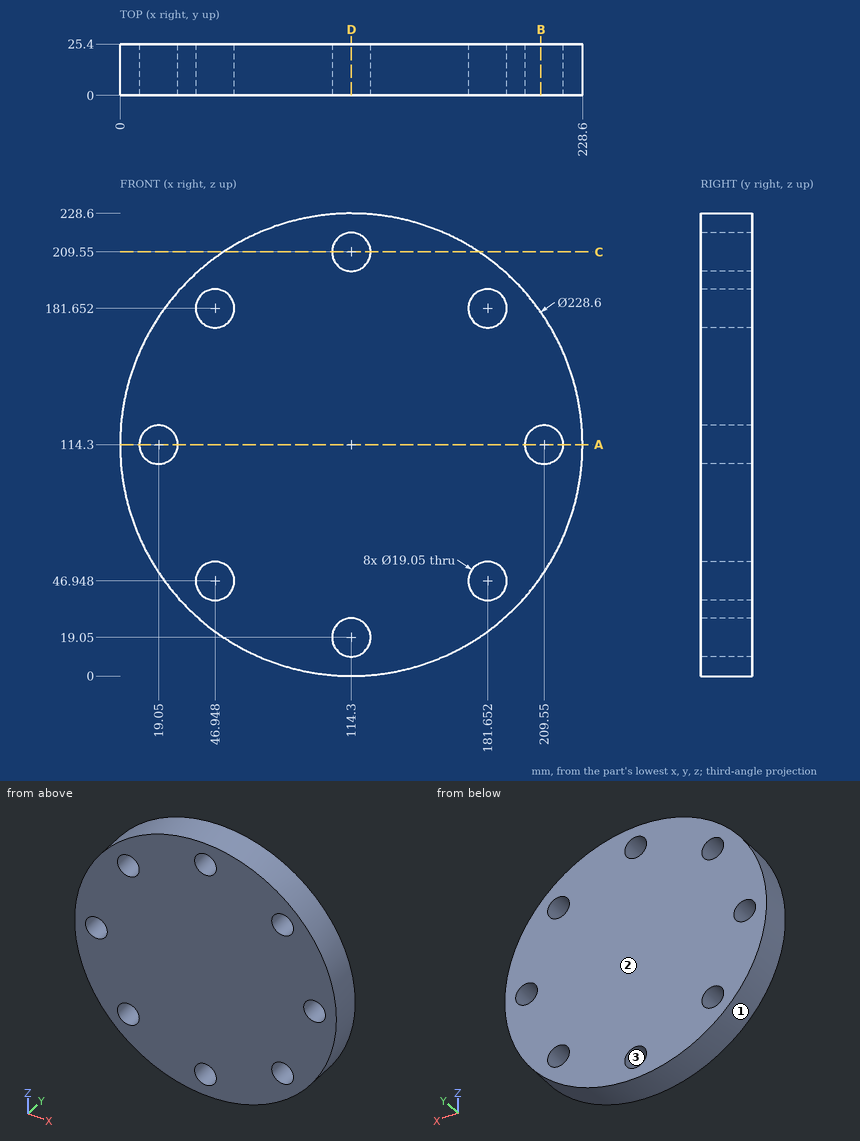
Study the drawing (mm; zero at the part's minimum x, y, z) and answer. Round coordinates to 2 decimals unless told otherwise and drop trailing zeros. Order: outer loops, then holes, each group sorted by start corner. A loop starts at its lowest first (then second) coordinate and runs counter-clockwise, first axis right, second up. Notation, with made-up numbers: M 67,60.25 L 83,60.25 A14 cw 83,82.25 Z; hole C 73,81 d1. An arc over 180 degrees is marked long. One line per item, written item: value.
Q1. Flat-ended cylindrical pins translate along their axes: pin 1 (4 mm diameter, centred on x = 174.5, z = 55.5, fed in from -Y); pin 2 (2 mm diameter, centred on x = 90.5, y = 17.5, fed in from +Z); pin 3 (4 mm diameter, centred on y = 8, z = 152, fed in from +X); pin 4 (10 mm diameter, centred on y = 10, z = 128.5, fed in from -X). Find the tip coordinate at first contact, or state that the pin passes through.
Derived:
pin 1: y = 0
pin 2: z = 226.3
pin 3: x = 222.88
pin 4: x = 0.37
Q2. Straight lines are drawn through the part: line 1 (Z direction, x = 114.3, y = 5.75) (3 decimals); line 2 (Z direction, x = 176, y = 14) (1 decimal); line 3 (X direction, y = 14, z = 212) (1 decimal). For each, find the intervals that lie inside material, in ascending order.
Derived:
line 1: 0 to 9.525, 28.575 to 200.025, 219.075 to 228.6
line 2: 18.1 to 39.3, 54.6 to 174, 189.3 to 210.5
line 3: 55 to 105.1, 123.5 to 173.6
Q3. Find section C-C on z = 209.55. Write down the section's boundary in (x, y) (3 decimals).
Derived:
outline: M 51.118,0 L 104.775,0 L 104.775,25.4 L 51.118,25.4 Z; M 123.825,0 L 177.482,0 L 177.482,25.4 L 123.825,25.4 Z
Q4. Determine the mould class of the marked faces 1, 2 and 3 for opening direction X: released by +X, released by -X, zero draft, split by the parting line, or undercut.
Derived:
face 1: split by the parting line
face 2: zero draft
face 3: undercut
Q5. Find section D-D on x = 114.3. Write down the section's boundary in (y, z) (3 decimals), then the cut area to 3 significant figures.
Derived:
outline: M 0,0 L 25.4,0 L 25.4,9.525 L 0,9.525 Z; M 0,28.575 L 25.4,28.575 L 25.4,200.025 L 0,200.025 Z; M 0,219.075 L 25.4,219.075 L 25.4,228.6 L 0,228.6 Z
area: 4,840 mm²
Q6. Find section B-B on x = 208. Write down the section's boundary in (y, z).
Derived:
outline: M 0,48.84 L 25.4,48.84 L 25.4,104.9 L 0,104.9 Z; M 0,123.7 L 25.4,123.7 L 25.4,179.76 L 0,179.76 Z
Q7. Find section A-A on z = 114.3. Write down the section's boundary in (x, y) (3 decimals).
Derived:
outline: M 0,0 L 9.525,0 L 9.525,25.4 L 0,25.4 Z; M 28.575,0 L 200.025,0 L 200.025,25.4 L 28.575,25.4 Z; M 219.075,0 L 228.6,0 L 228.6,25.4 L 219.075,25.4 Z
